Source: CAD feature listing. Evaluate the final solid. Frame: model axes, mm. A direction names the side the tool comes from. Give positions to 0.01 mm unless a question says otherwise; leave off trailing zeros. Order: outer loops, then holes, each group sorted by start corner. A loop starts at its lowest first (then second) coordinate and runs counter-clockwise, first axis right, second up.
```python
from build123d import *

# Parameters (mm, degrees)
SKETCH_1_W               = 36
SKETCH_1_H               = 36
EXTRUDE_1_DEPTH          = 10
SKETCH_2_W               = 24.56
SKETCH_2_H               = 24.56
EXTRUDE_2_DEPTH          = 2.5
SKETCH_3_R               = 6
EXTRUDE_3_DEPTH          = 12
SKETCH_4_R               = 7
EXTRUDE_4_DEPTH          = 6
CUT_EXTRUDE_START        = -0.5
SKETCH_5_R               = 6
CUT_EXTRUDE_1_DEPTH      = 0.5
SKETCH_7_R               = 6.5
EXTRUDE_5_DEPTH          = 0.3
CUT_EXTRUDE_2_REACH      = 48.595
CUT_EXTRUDE_2_END_RADIUS = 6.5
SKETCH_10_R              = 1
CUT_EXTRUDE_3_DEPTH      = 3
SKETCH_11_W              = 36.1
SKETCH_11_H              = 36.1
EXTRUDE_6_DEPTH          = 1
SKETCH_12_W              = 11
SKETCH_12_H              = 5
CUT_EXTRUDE_4_DEPTH      = 5


with BuildPart() as part:
    # 草图1 → 凸台-拉伸1 (new body)
    with BuildSketch(Plane.XY):
        Rectangle(SKETCH_1_W, SKETCH_1_H)
    extrude(amount=EXTRUDE_1_DEPTH)

    # 草图2 → 凸台-拉伸2 (add)
    with BuildSketch(Plane.XY.offset(10)):
        Rectangle(SKETCH_2_W, SKETCH_2_H)
    extrude(amount=EXTRUDE_2_DEPTH)

    # 草图3 → 凸台-拉伸3 (add)
    with BuildSketch(Plane.XY.offset(12.5)):
        Circle(SKETCH_3_R)
    extrude(amount=EXTRUDE_3_DEPTH)

    # 草图4 → 凸台-拉伸4 (add)
    with BuildSketch(Plane.XY.offset(24.5)):
        Circle(SKETCH_4_R)
    extrude(amount=EXTRUDE_4_DEPTH)

    # 草图5 → 切除-拉伸1 (cut)
    with BuildSketch(Plane.XY.offset(30.5).offset(CUT_EXTRUDE_START)):
        Circle(SKETCH_5_R)
    extrude(amount=CUT_EXTRUDE_1_DEPTH, mode=Mode.SUBTRACT)

    # 草图7 → 凸台-拉伸5 (add)
    with BuildSketch(Plane.XY.offset(12.5)):
        with Locations(Location((0, 0, 0), (0, 0, 180))):
            Circle(SKETCH_7_R)
    extrude(amount=EXTRUDE_5_DEPTH)

    # 切除-拉伸2: up to this cylinder (the profile starts outside it)
    cut_extrude_2_end = Plane(origin=(0, 0, 11.416503), z_dir=(0, 0, -1)) * Cylinder(CUT_EXTRUDE_2_END_RADIUS, 111.19, mode=Mode.PRIVATE)
    # 草图9 → 切除-拉伸2 (cut, up to the surface)
    with BuildSketch(Plane(origin=(12.28, 0, 0), x_dir=(0, 0, -1), z_dir=(1, 0, 0)), mode=Mode.PRIVATE) as cut_extrude_2_sk1:
        with BuildLine():
            Line((-10, -1.020232895), (-10, 1.020232895))
            ThreePointArc((-10, 1.020232895), (-10.939857211, 2.52041951), (-12.5, 3.35698746))
            Line((-12.5, 3.35698746), (-12.5, -3.35698746))
            ThreePointArc((-12.5, -3.35698746), (-10.939857211, -2.52041951), (-10, -1.020232895))
        make_face()
    cut_extrude_2_tool1 = extrude(cut_extrude_2_sk1.sketch, amount=-CUT_EXTRUDE_2_REACH, mode=Mode.PRIVATE) - cut_extrude_2_end
    add(cut_extrude_2_tool1.solids().sort_by_distance((12.28, 0, 11.416503))[0], mode=Mode.SUBTRACT)

    # 草图10 → 切除-拉伸3 (cut)
    with BuildSketch(Plane(origin=(18, 0, 0), x_dir=(0, 0, -1), z_dir=(1, 0, 0))):
        with Locations((-5, 0)):
            Circle(SKETCH_10_R)
    cut_extrude_3 = extrude(amount=-CUT_EXTRUDE_3_DEPTH, mode=Mode.SUBTRACT)

    # 镜向1: 切除-拉伸3 across plane
    add(cut_extrude_3.mirror(Plane(origin=(0, 0, 0), x_dir=(0, 0, 1), z_dir=(1, 0, 0))), mode=Mode.SUBTRACT)

    # 草图11 → 凸台-拉伸6 (add)
    with BuildSketch(Plane(origin=(0, 0, 0), x_dir=(-1, 0, 0), z_dir=(0, 0, -1))):
        Rectangle(SKETCH_11_W, SKETCH_11_H)
    extrude(amount=EXTRUDE_6_DEPTH)

    # 草图12 → 切除-拉伸4 (cut)
    with BuildSketch(Plane(origin=(0, 0, -1), x_dir=(-1, 0, 0), z_dir=(0, 0, -1))):
        with Locations((0, -13.05)):
            Rectangle(SKETCH_12_W, SKETCH_12_H)
    extrude(amount=-CUT_EXTRUDE_4_DEPTH, mode=Mode.SUBTRACT)


solid = part.part
```
1) Draft query along Z for faces 1 (the flat face through (-2, 6, 12.8)), 2 (the flat face through (6, 2, 30.5)), 3 (the flat face through (0.3, -18.05, -0.5)). Return one class per face: +Z half, -Z half, draft (parallel to the pull), parting line (faces both ways), or undercut.
Report:
face 1: undercut
face 2: +Z half
face 3: draft
2) Material intervals for L1, parallel to Y at x = 16.4, z = 5; L2, parallel to Y at x = -4.5, z = 1.5; L3, parallel to Z at x = -7, y = 12, sorted ascending.
Report:
L1: y = -18 to -1, 1 to 18
L2: y = -18 to -15.55, -10.55 to 18
L3: z = -1 to 12.5
3) Section query A-A, the plane x = 15.5. Return the cut outline in (y, z), and give its area (3 significant figures).
Report:
outline: (-18.05, -1) - (18.05, -1) - (18.05, 0) - (18, 0) - (18, 10) - (-18, 10) - (-18, 0) - (-18.05, 0) - close; hole circle Ø2 at (0, 5)
area: 393 mm2
4) Section query B-B, the plane z = 2.5. Return the cut outline in (x, y), and give its area (3 significant figures).
Report:
outline: (-18, -18) - (18, -18) - (18, 18) - (-18, 18) - close; hole (-5.5, -15.55) - (5.5, -15.55) - (5.5, -10.55) - (-5.5, -10.55) - close
area: 1,240 mm2
5) Pin query (flat end, axial travel): pin 1 (5 mm diameter, centred on x = 7, y = 8, fed in from +Z); pin 2 (1.8 mm diameter, centred on y = 0, z = 5, fed in from -X); pin 3 (12 mm diameter, centred on y = 10.5, z = 14.5, fed in from -X). Return the tip coordinate at first contact, or that it passes through.
Report:
pin 1: stops at z = 12.5
pin 2: stops at x = -15
pin 3: stops at x = -18
6) Reachability of faces 4 (the flat face through (0, 12.28, 11)), 5 (the cylindrical face through (-16.5, -0.6, 5.8)), 6 (the flat face through (5.5, -13, 1)) from +Z, -Z, +X, -X, +Y, -Y: full face, straight path, thin tool, end or side. Return the list, or none.
Report:
face 4: +Z, +X, -X, +Y
face 5: -X
face 6: -Z
